from build123d import *

# Parameters (mm, degrees)
F1_DEPTH = 77
F2_DEPTH = 5
F3_SIZE  = 42
F4_R     = 5
F5_DEPTH = 1000
F7_DEPTH = 10000


with BuildPart() as f1:
    # F0 (on Top) → F1 (new body)
    with BuildSketch(Plane.XY):
        Polygon((-53.768117, 18.507083), (-53.768117, -56.492917), (1.731883, -56.492917), (57.231883, -56.492917), (57.231883, -30.815218), (57.231883, 18.507083), (52.231883, 18.507083), (-48.768117, 18.507083), align=None)
        with BuildLine():
            ThreePointArc((7.731883, -31.492917), (5.974524, -35.735557), (1.731883, -37.492917))
            ThreePointArc((1.731883, -37.492917), (-2.510758, -27.250276), (7.731883, -31.492917))
        make_face(mode=Mode.SUBTRACT)
    extrude(amount=F1_DEPTH)

    # F0 (on Top) → F2 (join)
    with BuildSketch(Plane.XY):
        Polygon((-48.768117, 73.507083), (-48.768117, 18.507083), (52.231883, 18.507083), (52.231883, 73.507083), (23.231883, 73.507083), (-19.768117, 73.507083), align=None)
        with BuildLine():
            ThreePointArc((-13.768117, 48.507083), (-24.010758, 44.264443), (-19.768117, 54.507083))
            ThreePointArc((-19.768117, 54.507083), (-15.525476, 52.749724), (-13.768117, 48.507083))
        make_face(mode=Mode.SUBTRACT)
        with BuildLine():
            ThreePointArc((29.231883, 48.507083), (18.989242, 44.264443), (23.231883, 54.507083))
            ThreePointArc((23.231883, 54.507083), (27.474524, 52.749724), (29.231883, 48.507083))
        make_face(mode=Mode.SUBTRACT)
    extrude(amount=F2_DEPTH)

    # F3
    f3_edges = [f1.edges().sort_by_distance(p)[0] for p in [
        (1.731883, 18.507083, 77),
    ]]
    chamfer(f3_edges, length=F3_SIZE)

    # F4 (on face) → F5 (cut)
    with BuildSketch(Plane(origin=(-53.768117, 0, 0), x_dir=(0, -1, 0), z_dir=(-1, 0, 0))):
        with Locations((31.492917, 27)):
            Circle(F4_R)
        with Locations((31.492917, 62)):
            Circle(F4_R)
    extrude(amount=-F5_DEPTH, mode=Mode.SUBTRACT)

    # F6 (on face) → F7 (cut)
    with BuildSketch(Plane.XZ.offset(56.492917)):
        with BuildLine():
            Line((52.231883, 77), (-48.768117, 77))
            Line((-48.768117, 77), (-48.768117, 8))
            ThreePointArc((-48.768117, 8), (-47.889437, 5.87868), (-45.768117, 5))
            Line((-45.768117, 5), (49.231883, 5))
            ThreePointArc((49.231883, 5), (51.353203, 5.87868), (52.231883, 8))
            Line((52.231883, 8), (52.231883, 77))
        make_face()
    extrude(amount=-F7_DEPTH, mode=Mode.SUBTRACT)


solid = f1.part
Geometry: final body of the model. Coordinates: model frame, mm. A direction names the side the tool comes from. Round coordinates to 2 decimals unless told otherwise and drop trailing zeros. Write each loop counter-clockwise with the first axis right and the second up, starting at its lowest first coordinate (ties: lowest second). Pieces come first, ordered by that corner, then holes. Notation, with made-up numbers: M -35,52.5 L 6,52.5 A26 cw 6,85.5 Z; hole C 4,60.5 d4. An arc over 180 degrees is marked long. Write item = value, one per line.
Item 1: Pull-direction query (X, two-part tool) for faces 1 (the face through (52.232, 46, 2)), 2 (the face through (1, 9, 5)), 3 (the face through (-53.768, -18, 29)), 4 (the face through (54, 18.507, 17)); classes: pulls with the +X half, pulls with the -X half, needs draft (parallel to the pull), parting line crosses it, or undercut.
Findings:
face_1 = pulls with the +X half
face_2 = undercut
face_3 = pulls with the -X half
face_4 = needs draft
Item 2: Pin query (flat end, axial travel): P1, Ø15.5, axis at x = -19.77, y = 48.51, coming from the +Z side; P2, Ø2.5, axis at x = 55, z = 22, coming from the +Y side; P3, Ø1.5, axis at y = 53, z = 2, coming from the +X side. Return the tip coordinate at first contact, or that it passes through.
Findings:
P1 = 5
P2 = 18.51
P3 = 52.23
Item 3: Section query A-A on z = 17. Return loops of the section in (x, y), then the cut area to 3 significant figures.
Findings:
outline = M -53.77,-56.49 L -48.77,-56.49 L -48.77,18.51 L -53.77,18.51 Z; M 52.23,-56.49 L 57.23,-56.49 L 57.23,18.51 L 52.23,18.51 Z
area = 750 mm^2
Item 4: Section query D-D on y = -28. State how many separate pieces and enclosed holes the cut face has, then the cut area to 3 significant figures.
Findings:
separate_pieces = 6
enclosed_holes = 0
area = 1,090 mm^2
Item 5: Section query B-B on z = 27. Return loops of the section in (x, y).
Findings:
outline = M -53.77,-56.49 L -48.77,-56.49 L -48.77,-36.49 L -53.77,-36.49 Z; M -53.77,-26.49 L -48.77,-26.49 L -48.77,18.51 L -53.77,18.51 Z; M 52.23,-56.49 L 57.23,-56.49 L 57.23,-36.49 L 52.23,-36.49 Z; M 52.23,-26.49 L 57.23,-26.49 L 57.23,18.51 L 52.23,18.51 Z
Item 6: Material intervals for line 1 along X through (y, z) = (-24, 41); line 2 along Z through (x, y) = (-10, -2), sorted ascending. Write a range as [from, to].
Findings:
line_1 = [-53.77, -48.77], [52.23, 57.23]
line_2 = [0, 5]
Item 7: Section query C-C on x = 25. Return loops of the section in (y, z), then the cut area to 3 significant figures.
Findings:
outline = M -56.49,0 L 42.77,0 L 42.77,5 L -56.49,5 Z; M 54.24,0 L 73.51,0 L 73.51,5 L 54.24,5 Z
area = 593 mm^2
Item 8: Access query for faces 5 (the face through (55, -40, 77)), 6 (the face through (52.232, -28, 34)), 7 (the face through (-48.768, 46, 2)). Directions: +Z, -Z, +X, -X, +Y, -Y. A direction counts if a zero-diameter tool reaches every point of the face in a straight line with its end or side. Return the directions, or none.
Findings:
face_5 = +Z, +X, -X, +Y, -Y
face_6 = +Z, +Y, -Y
face_7 = +Z, -Z, -X, +Y
